Input: part model. Units: mm. Frame: model coordinates. Round coordinates to 2 decimals unless told otherwise and drop trailing zeros. Loops run counter-clockwise (first coordinate to the right, second up) from the corner with the lowest first, then second, coordinate; pieces in that order, holes last. Notation, with made-up numbers: M 18,59.25 L 55,59.25 A33 ccw 55,87.25 Z; hole C -22.5,61 d11. An arc over 180 degrees is marked long. Put each result on its own line as item: value. Start each with the question number.
1) Section D-D on x = -47. Output: boundary loops of the cut face in (y, z).
2) Line query: probe 1 along X at (y, z) = (-3, 1.8); probe 2 along Y at (x, z) = (-60.5, 1.95); probe 3 along X at (y, z) = (-8.5, 2.35). Output: solid intervals per line, ascending.
3) Section A-A on z = 1.2. Output: boundary loops of the cut face in (x, y), plus the area to 3 significant figures.
4) Section C-C on y = -2. Output: boundary loops of the cut face in (x, z).
5) Pin query (flat end, axial travel): pin 1 (0.9 mm diameter, centred on y = -11, z = 1.5, fed in from +X); pin 2 (1.5 mm diameter, centred on x = -154.5, z = 2, fed in from -Y). Return the tip coordinate at first contact, or that it passes through.
6) Section B-B on y = -17. Output: boundary loops of the cut face in (x, z), plus the area to 3 significant figures.
from build123d import *

# Parameters (mm, degrees)
SKETCH1_R           = 2.5
BOSS_EXTRUDE1_DEPTH = 3
BOSS_EXTRUDE2_START = -3
SKETCH3_R           = 22.5
SKETCH3_R_2         = 5
BOSS_EXTRUDE2_DEPTH = 3


with BuildPart() as part:
    # Sketch1 → Boss-Extrude1 (new body)
    # profile 1 of 8: a face of its own
    with BuildSketch(Plane.XY):
        with BuildLine():
            ThreePointArc((22.5, 0), (15.909902577, 15.909902577), (0, 22.5))
            Line((0, 22.5), (-22.5, 0))
            Line((-22.5, 0), (-22.124973736, -4.090909091))
            ThreePointArc((-22.124973736, -4.090909091), (2.054031517, -22.406047276), (22.5, 0))
        make_face()
        with BuildLine():
            ThreePointArc((-7.5, 5), (-9.267766953, 9.267766953), (-5, 7.5))
            Line((-5, 7.5), (-5, 9))
            Line((-5, 9), (-2.405779746, 18.179870439))
            ThreePointArc((-2.405779746, 18.179870439), (0, 20), (2.405779746, 18.179870439))
            Line((2.405779746, 18.179870439), (5, 9))
            Line((5, 9), (5, 7.5))
            ThreePointArc((5, 7.5), (7.5, 10), (10, 7.5))
            ThreePointArc((10, 7.5), (9.267766953, 5.732233047), (7.5, 5))
            Line((7.5, 5), (9, 5))
            Line((9, 5), (18.179870439, 2.405779746))
            ThreePointArc((18.179870439, 2.405779746), (19.493699588, 1.508363998), (20, 0))
            ThreePointArc((20, 0), (19.493699588, -1.508363998), (18.179870439, -2.405779746))
            Line((18.179870439, -2.405779746), (9, -5))
            Line((9, -5), (7.5, -5))
            ThreePointArc((7.5, -5), (9.267766953, -5.732233047), (10, -7.5))
            ThreePointArc((10, -7.5), (7.5, -10), (5, -7.5))
            Line((5, -7.5), (5, -9))
            Line((5, -9), (2.405779746, -18.179870439))
            ThreePointArc((2.405779746, -18.179870439), (0, -20), (-2.405779746, -18.179870439))
            Line((-2.405779746, -18.179870439), (-5, -9))
            Line((-5, -9), (-5, -7.5))
            ThreePointArc((-5, -7.5), (-9.267766953, -9.267766953), (-7.5, -5))
            Line((-7.5, -5), (-9, -5))
            Line((-9, -5), (-18.179870439, -2.405779746))
            ThreePointArc((-18.179870439, -2.405779746), (-20, 0), (-18.179870439, 2.405779746))
            Line((-18.179870439, 2.405779746), (-9, 5))
            Line((-9, 5), (-7.5, 5))
        make_face(mode=Mode.SUBTRACT)
    # profile 2 of 8: a face of its own
    with BuildSketch(Plane.XY):
        with Locations((-7.5, 7.5)):
            Circle(SKETCH1_R)
    # profile 3 of 8: a face of its own
    with BuildSketch(Plane.XY):
        with Locations((7.5, 7.5)):
            Circle(SKETCH1_R)
    # profile 4 of 8: a face of its own
    with BuildSketch(Plane.XY):
        with Locations((7.5, -7.5)):
            Circle(SKETCH1_R)
    # profile 5 of 8: a face of its own
    with BuildSketch(Plane.XY):
        with Locations((-7.5, -7.5)):
            Circle(SKETCH1_R)
    # profile 6 of 8: a face of its own
    with BuildSketch(Plane.XY):
        Polygon((-22.5, 22.5), (0, 22.5), (-22.5, 0), align=None)
    # profile 7 of 8: a face of its own
    with BuildSketch(Plane.XY):
        Polygon((-22.5, 0), (-22.5, 22.5), (-162.5, 22.5), (-162.5, -11.5), (-137.5, -11.5), (-137.5, -26.5), (-117.5, -26.5), (-117.5, 0), align=None)
    # profile 8 of 8: a face of its own
    with BuildSketch(Plane.XY):
        with BuildLine():
            Line((-22.5, 0), (-22.124973736, -4.090909091))
            ThreePointArc((-22.124973736, -4.090909091), (-23.843623821, -1.156469426), (-27.041634566, 0))
            Line((-27.041634566, 0), (-22.5, 0))
        make_face()
    extrude(amount=BOSS_EXTRUDE1_DEPTH)

    # Sketch3 → Boss-Extrude2 (add)
    with BuildSketch(Plane.XY.offset(3).offset(BOSS_EXTRUDE2_START)):
        Circle(SKETCH3_R)
        Circle(SKETCH3_R_2, mode=Mode.SUBTRACT)
    extrude(amount=BOSS_EXTRUDE2_DEPTH)


solid = part.part
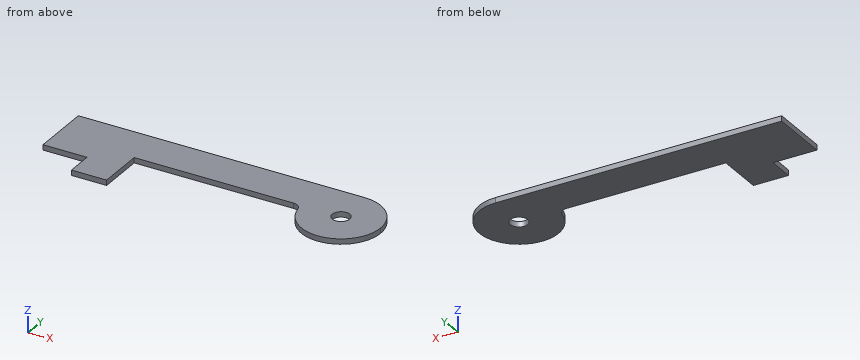
Geometry results:
1. outline: M 0,0 L 22.5,0 L 22.5,3 L 0,3 Z
2. probe 1: x = -162.5 to -117.5, -22.46 to -4, 4 to 22.3
2. probe 2: y = 0 to 22.5
2. probe 3: x = -162.5 to -117.5, -20.83 to 20.83
3. outline: M -162.5,-11.5 L -137.5,-11.5 L -137.5,-26.5 L -117.5,-26.5 L -117.5,0 L -27.04,0 A5 cw -22.12,-4.09 A22.5 ccw long 0,22.5 L -162.5,22.5 Z; hole C 0,0 d10
3. area: 5,590 mm²
4. outline: M -162.5,0 L -117.5,0 L -117.5,3 L -162.5,3 Z; M -23.04,0 L -4.58,0 L -4.58,3 L -23.04,3 Z; M 4.58,0 L 22.41,0 L 22.41,3 L 4.58,3 Z
5. pin 1: stops at x = 19.87
5. pin 2: stops at y = -11.5
6. outline: M -137.5,0 L -117.5,0 L -117.5,3 L -137.5,3 Z; M -14.74,0 L 14.74,0 L 14.74,3 L -14.74,3 Z
6. area: 148 mm²
